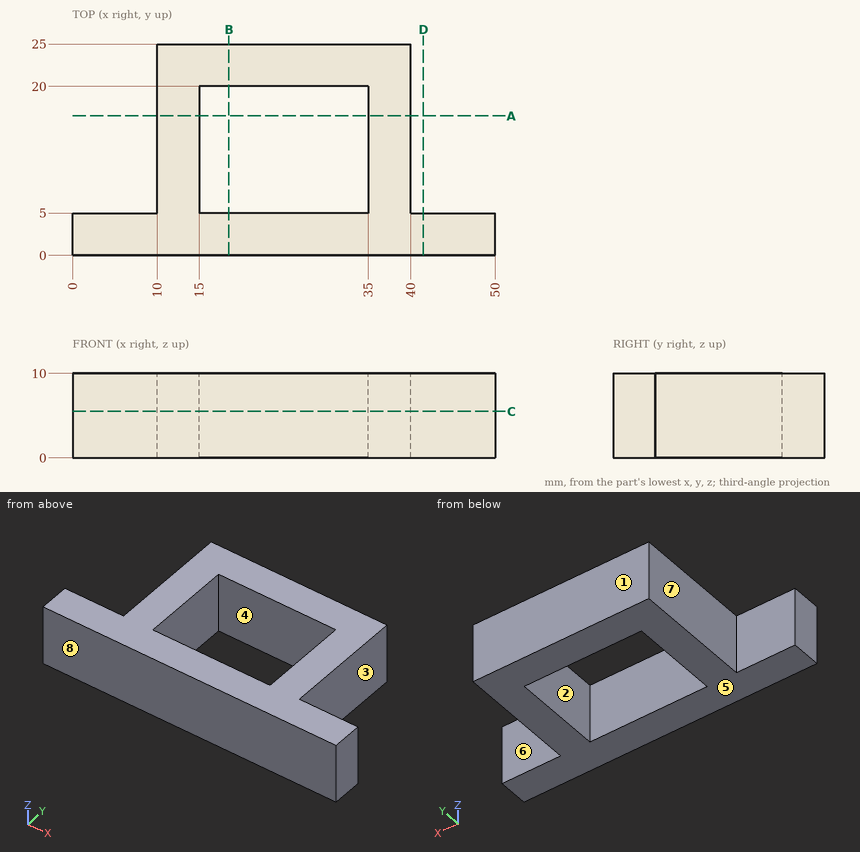
Geometry: see drawing. Coordinates: mm, zero at the bounding-box minimum. A direction names the side the tool comes from. Round coordinates to 2 decimals unless told otherwise and drop trailing zeros. Loops run counter-clockwise (first coordinate to the right, second up) from the corner with the lowest first, then second, coordinate; pieces in that order, holes last. Notation, with made-up numbers: (-31.5, 42) - (-12.5, 42) arc R17 cw to (-12.5, 51) - close; hole circle Ø8 at (36.25, 22). An arc over 180 degrees is marked (long way). Write item = value, one per line. Start each with the question number.
(1) Section query C-C, the plane z = 5.5. Output: boundary loops of the cut face in (x, y), plus the area to 3 significant figures.
(2) Ray query, line 1 along X through (y, z) = (10.75, 9.75); line 2 along Y through (x, z) = (24, 6.25); line 3 along X through (y, z) = (21, 2.5). Return the intervals inside material, ascending. Write a range as from..to.
(3) Section query B-B, the plane x = 18.5. Output: boundary loops of the cut face in (y, z), plus the area to 3 significant figures.
(4) Pin query (flat end, axial travel): pin 1 (12 mm diameter, centred on x = 17, y = 9.5, fed in from -Z); pin 2 (3 mm diameter, centred on y = 13.5, z = 6.5, fed in from -X); pin 3 (3 mm diameter, centred on y = 13.5, z = 4.5, fed in from +X); pin 4 (5 mm diameter, centred on x = 5, z = 7, fed in from +Y). Return the tip coordinate at first contact, or that it passes through.
(5) Section query D-D, the plane x = 41.5. Output: boundary loops of the cut face in (y, z).
(6) Section query A-A, the plane y = 16.5. Output: boundary loops of the cut face in (x, z).
(7) Pull-direction query (Y, two-part tool) for the marked faces 1, 2 and 3; classes: +Y half, -Y half, draft (parallel to the pull), parting line (faces both ways), or undercut.
(8) Set-up query: the marked faces 4, 5, 6, 7 and 8. Return all of +Z, -Z, +X, -X, +Y, -Y with unobstructed straight access to the full face (end or side cutting, diameter ignored); none if empty.
Conclusion:
q1.outline = (0, 0) - (50, 0) - (50, 5) - (40, 5) - (40, 25) - (10, 25) - (10, 5) - (0, 5) - close; hole (15, 5) - (35, 5) - (35, 20) - (15, 20) - close
q1.area = 550 mm2
q2.line_1 = 10..15, 35..40
q2.line_2 = 0..5, 20..25
q2.line_3 = 10..40
q3.outline = (0, 0) - (5, 0) - (5, 10) - (0, 10) - close; (20, 0) - (25, 0) - (25, 10) - (20, 10) - close
q3.area = 100 mm2
q4.pin_1 = 0
q4.pin_2 = 10
q4.pin_3 = 40
q4.pin_4 = 5
q5.outline = (0, 0) - (5, 0) - (5, 10) - (0, 10) - close
q6.outline = (10, 0) - (15, 0) - (15, 10) - (10, 10) - close; (35, 0) - (40, 0) - (40, 10) - (35, 10) - close
q7.face_1 = +Y half
q7.face_2 = undercut
q7.face_3 = draft
q8.face_4 = +Z, -Z
q8.face_5 = -Z, +X, -X, +Y, -Y
q8.face_6 = +Z, -Z, +X, +Y
q8.face_7 = +Z, -Z, -X, +Y
q8.face_8 = +Z, -Z, +X, -X, -Y
